Source: CAD feature listing. Evaluate the final solid. Frame: model axes, mm. A direction names the side the tool comes from. Round coordinates to 2 decimals unless told otherwise and drop trailing zeros. Order: outer loops, then holes, each group sorted by start corner. A loop starts at its lowest first (then second) coordinate and runs counter-clockwise, first axis right, second up. Notation, with made-up numbers: (-19.5, 29) -> (0.5, 29) arc R19 ccw to (0.5, 54) -> close; hole circle Ø8 at (77.25, 67). An arc over 180 degrees is marked (long way). One line per item, written item: value. Start each with the question number.
1) Section A-A (y = 1). Return the cut outline in (x, z), and give its area (3 significant figures).
2) Section B-B (x = 14). Return the cut outline in (y, z), and give its area (3 significant figures).
3) Reachability of faces 1 (the face through (19.5, 3, 0)), 2 (the face through (15, -4, 0)), 3 (the face through (2, 0.8, 5.2)), 4 (the face through (2, 0.4, -5.2)), 5 (the face through (15, 4, 0)) from +Z, -Z, +X, -X, +Y, -Y: full face, straight path, thin tool, end or side. Return the list, or none.
4) Ray query, L1, parallel to Y at x = 14.5, z = 0; L2, parallel to Y at x = 4.75, z = 0; L3, parallel to Z at x = 17.5, y = -3. Return the intervals inside material, ascending.
5) Section C-C (z = 1.25). Return the cut outline in (x, y), and give its area (3 significant figures).
6) Mould query, pull axis Z, two halves, no side actions, for faces 6 (the face through (1, 0.1, -6.5)), 7 (the face through (10, -4.4, 0)), 8 (the face through (11, -3, -4)), 9 (the face through (9.89, -2.44, 0.54)). Classes: pulls with the +Z half, pulls with the -Z half, needs draft (parallel to the pull), parting line crosses it, or undercut.
7) Pin query (flat end, axial travel): P1, Ø4, axis at x = 12, y = -2, coming from the -Z side; P2, Ø1.5, axis at x = 13.5, y = -1.5, coming from the -Z side; P3, Ø5, axis at x = 17, z = -0.5, coming from the -Y side. Return the tip coordinate at first contact, or that it passes through.
```python
from build123d import *

# Parameters (mm, degrees)
SKETCH1_W           = 8.306623862
SKETCH1_H           = 10
BOSS_EXTRUDE1_DEPTH = 2
SKETCH2_R           = 5
BOSS_EXTRUDE2_DEPTH = 8
SKETCH3_W           = 6
SKETCH3_H           = 8
BOSS_EXTRUDE3_DEPTH = 9.5
SKETCH4_R           = 2.5
CUT_EXTRUDE1_DEPTH  = 20.5


with BuildPart() as part:
    # Sketch1 → Boss-Extrude1 (new body)
    with BuildSketch(Plane(origin=(0, 0, 0), x_dir=(0, 0, -1), z_dir=(1, 0, 0))):
        with BuildLine():
            Line((-4.153311931, -5), (-4.153311931, 5))
            ThreePointArc((-4.153311931, 5), (-6.5, 0), (-4.153311931, -5))
        make_face()
        Rectangle(SKETCH1_W, SKETCH1_H)
        with BuildLine():
            Line((4.153311931, -5), (4.153311931, 5))
            ThreePointArc((4.153311931, 5), (6.5, 0), (4.153311931, -5))
        make_face()
    extrude(amount=BOSS_EXTRUDE1_DEPTH)

    # Sketch2 → Boss-Extrude2 (add)
    with BuildSketch(Plane(origin=(2, 0, 0), x_dir=(0, 0, -1), z_dir=(1, 0, 0))):
        Circle(SKETCH2_R)
    extrude(amount=BOSS_EXTRUDE2_DEPTH)

    # Sketch3 → Boss-Extrude3 (add)
    with BuildSketch(Plane(origin=(10, 0, 0), x_dir=(0, 0, -1), z_dir=(1, 0, 0))):
        with BuildLine():
            ThreePointArc((-3, 4), (-5, 0), (-3, -4))
            Line((-3, -4), (-3, 4))
        make_face()
        Rectangle(SKETCH3_W, SKETCH3_H)
        with BuildLine():
            Line((3, 4), (3, -4))
            ThreePointArc((3, -4), (4.472135955, -2.236067977), (5, 0))
            ThreePointArc((5, 0), (4.472135955, 2.236067977), (3, 4))
        make_face()
    extrude(amount=BOSS_EXTRUDE3_DEPTH)

    # Sketch4 → Cut-Extrude1 (cut, through all)
    with BuildSketch(Plane(origin=(19.5, 0, 0), x_dir=(0, 0, -1), z_dir=(1, 0, 0))):
        Circle(SKETCH4_R)
    extrude(amount=-CUT_EXTRUDE1_DEPTH, mode=Mode.SUBTRACT)


solid = part.part
```
Findings:
1. outline: (0, -6.42) -> (2, -6.42) -> (2, -4.9) -> (19.5, -4.9) -> (19.5, -2.29) -> (0, -2.29) -> close; (0, 2.29) -> (19.5, 2.29) -> (19.5, 4.9) -> (2, 4.9) -> (2, 6.42) -> (0, 6.42) -> close
1. area: 108 mm2
2. outline: (-4, -3) arc R5 ccw to (4, -3) -> (4, 3) arc R5 ccw to (-4, 3) -> close; hole circle Ø5 at (0, 0)
2. area: 50.7 mm2
3. face 1: +Z, -Z, +X, +Y, -Y
3. face 2: +Z, -Z, +X, -Y
3. face 3: +Z, +X
3. face 4: -Z, +X
3. face 5: +Z, -Z, +X, +Y
4. L1: -4 to -2.5, 2.5 to 4
4. L2: -5 to -2.5, 2.5 to 5
4. L3: -4 to 4
5. outline: (0, -5) -> (2, -5) -> (2, -4.84) -> (10, -4.84) -> (10, -4) -> (19.5, -4) -> (19.5, -2.17) -> (0, -2.17) -> close; (0, 2.17) -> (19.5, 2.17) -> (19.5, 4) -> (10, 4) -> (10, 4.84) -> (2, 4.84) -> (2, 5) -> (0, 5) -> close
5. area: 89.0 mm2
6. face 6: pulls with the -Z half
6. face 7: needs draft
6. face 8: parting line crosses it
6. face 9: undercut
7. P1: z = -5
7. P2: z = -4.94
7. P3: y = -4
